The listing builds one solid part. Answer for the finished solid, in the listing's coordinates (mm). Face numbers are marked on the shaded views. Give positions to 0.01 mm unless a question says otherwise; leave off trailing zeros. Write each loop counter-clockwise with the first axis right and the second up, starting at its lowest first coordinate (ties: lowest second). Pieces come first, ordered by that corner, then holes. Notation, with made-up numbers: (19.5, -37) - (58.5, -37) arc R28 cw to (58.5, -4) - close; hole circle Ø7 at (-35, 10.25). An arc over 180 degrees is marked (long way). Answer as CSV lines item,"result". Start each with the question number.
(1) Find section C-C (z = -15). Write down the section's boundary in (x, y), then the cut area to 3 significant figures.
(2) Find section B-B (x = 2). Write down the section's boundary in (y, z).
(3) For a pull along Y with two mould halves and no side action, classify the marked faces 1, 2 and 3 as pulls with the +Y half, pulls with the -Y half, needs draft (parallel to the pull), parting line crosses it, or undercut.
(4) Straight lines are drawn through the part: probe 1 along X at (y, z) = (-27.5, -10); probe 2 along Y at (x, z) = (8, -9); probe 3 along Y at (x, z) = (-6.5, -25). For each, find the intervals that lie inside material, in ascending order.
(5) Find section D-D (y = -24). Write down the section's boundary in (x, z), then the cut area to 3 significant figures.
(6) Find section A-A (y = -37). Write down the section's boundary in (x, z), then the cut area to 3 significant figures.
from build123d import *

# Parameters (mm, degrees)
F0_W     = 57.621952
F0_H     = 59.63415
F1_DEPTH = 50
F3_D     = 25
F4_R     = 4


with BuildPart() as f1:
    # F0 (on Front) → F1 (new body)
    with BuildSketch(Plane.XZ):
        Rectangle(F0_W, F0_H)
    extrude(amount=F1_DEPTH)

    # F3 (through all)
    with Locations(Plane(origin=(0, 0, -29.817075), x_dir=(1, 0, 0), z_dir=(0, 0, -1))):
        with Locations((-2.286586, 27.2561)):
            Hole(F3_D / 2)

    # F4
    f4_edges = [f1.edges().sort_by_distance(p)[0] for p in [
        (0, -50, -29.817075),
        (-28.810976, -50, 0),
        (0, -50, 29.817075),
        (28.810976, -50, 0),
    ]]
    fillet(f4_edges, radius=F4_R)


solid = f1.part
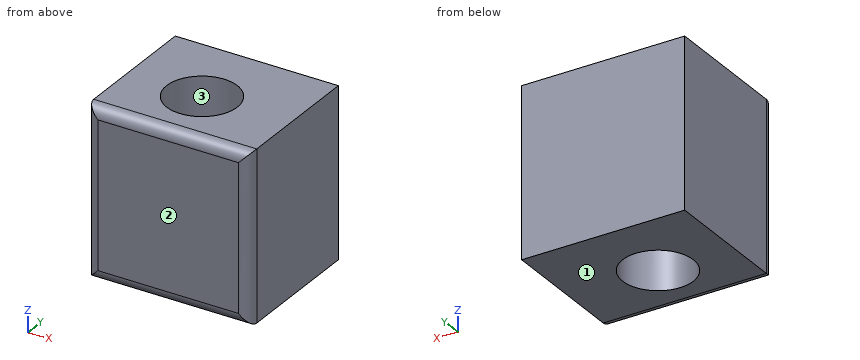
Result set:
1,outline,"(-28.81, -46) arc R4 ccw to (-24.81, -50) - (24.81, -50) arc R4 ccw to (28.81, -46) - (28.81, 0) - (-28.81, 0) - close; hole circle Ø25 at (-2.29, -27.26)"
1,area,"2,380 mm^2"
2,outline,"(-50, -25.82) arc R4 ccw to (-46, -29.82) - (-39, -29.82) - (-39, 29.82) - (-46, 29.82) arc R4 ccw to (-50, 25.82) - close; (-15.51, -29.82) - (0, -29.82) - (0, 29.82) - (-15.51, 29.82) - close"
3,face 1,"needs draft"
3,face 2,"pulls with the -Y half"
3,face 3,"undercut"
4,probe 1,"-28.81 to -14.78, 10.21 to 28.81"
4,probe 2,"-50 to -34.36, -20.15 to 0"
4,probe 3,"-50 to -39.02, -15.49 to 0"
5,outline,"(-28.81, -29.82) - (-14.36, -29.82) - (-14.36, 29.82) - (-28.81, 29.82) - close; (9.78, -29.82) - (28.81, -29.82) - (28.81, 29.82) - (9.78, 29.82) - close"
5,area,"2,000 mm^2"
6,outline,"(-28.81, -29.82) - (-10.12, -29.82) - (-10.12, 29.82) - (-28.81, 29.82) - close; (5.54, -29.82) - (28.81, -29.82) - (28.81, 29.82) - (5.54, 29.82) - close"
6,area,"2,500 mm^2"
